```python
from build123d import *

# Parameters (mm, degrees)
SKETCH1_R                   = 6.8
SKETCH1_R_2                 = 4.8
TUBE_SURROUNDING_DEPTH      = 50
FIN_START                   = -100
FIN_HOLDERS_DEPTH           = 100
F_3MM_SUPPORT_FILLETS_R     = 3
F_5MM_FIN_HOLDER_ROUNDING_R = 5


with BuildPart() as part:
    # Sketch1 → Tube surrounding (new, symmetric)
    with BuildSketch(Plane.XY):
        Circle(SKETCH1_R)
        Circle(SKETCH1_R_2, mode=Mode.SUBTRACT)
    extrude(amount=TUBE_SURROUNDING_DEPTH, both=True)

    # Sketch2 → Fin holders (add)
    with BuildSketch(Plane.XY.offset(50).offset(FIN_START)):
        with BuildLine():
            Line((-6.239343856, 2.70380995), (-2.70380995, 6.239343856))
            Line((-2.70380995, 6.239343856), (-8.3606642, 11.896198106))
            Line((-8.3606642, 11.896198106), (-7.300004028, 12.956858277))
            Line((-7.300004028, 12.956858277), (0, 5.656854249))
            Line((0, 5.656854249), (7.300004028, 12.956858277))
            Line((7.300004028, 12.956858277), (8.3606642, 11.896198106))
            Line((8.3606642, 11.896198106), (2.70380995, 6.239343856))
            Line((2.70380995, 6.239343856), (6.239343856, 2.70380995))
            Line((6.239343856, 2.70380995), (11.896198106, 8.3606642))
            Line((11.896198106, 8.3606642), (12.956858277, 7.300004028))
            Line((12.956858277, 7.300004028), (4.704593429, -0.952260821))
            ThreePointArc((4.704593429, -0.952260821), (0, 4.8), (-4.704593429, -0.952260821))
            Line((-4.704593429, -0.952260821), (-12.956858277, 7.300004028))
            Line((-12.956858277, 7.300004028), (-11.896198106, 8.3606642))
            Line((-11.896198106, 8.3606642), (-6.239343856, 2.70380995))
        make_face()
    extrude(amount=FIN_HOLDERS_DEPTH)

    # 3mm support fillets
    # the kernel refuses this fillet: 3 mm, written as the material it adds along each edge
    with BuildSketch(Plane(origin=(1.060017294, 6.716871544, -50), x_dir=(-0.9973250573829818, 0.07309398002593596, 0), z_dir=(0, 0, 1)), Plane(origin=(-6.716871544, 1.060017294, -50), x_dir=(-0.07309398002594036, -0.9973250573829815, 0), z_dir=(0, 0, 1))) as f_3mm_support_fillets_piece_1:
        with BuildLine():
            CenterArc((1.38224034, -2.989581697), F_3MM_SUPPORT_FILLETS_R, 94.776406165, 44.415308597)
            Line((-0.88846134, -1.028991511), (0, 0))
            ThreePointArc((0, 0), (0.566218934, -0.023614819), (1.132437869, 0))
        make_face()
    extrude(amount=100)
    with BuildSketch(Plane(origin=(-1.060017294, 6.716871544, -50), x_dir=(-0.7071067811865461, 0.707106781186549, 0), z_dir=(0, 0, 1)), Plane(origin=(6.716871544, 1.060017294, -50), x_dir=(0.7071067811865486, 0.7071067811865466, 0), z_dir=(0, 0, 1))) as f_3mm_support_fillets_piece_2:
        with BuildLine():
            CenterArc((1.359480446, -3), F_3MM_SUPPORT_FILLETS_R, 90, 44.415308597)
            ThreePointArc((-0.740082191, -0.857142857), (-0.352167026, -0.444004423), (0, 0))
            Line((0, 0), (1.359480446, 0))
        make_face()
    extrude(amount=100)

    # 5mm fin holder rounding
    # the kernel refuses this fillet: 5 mm, written as the material it takes off along each edge
    with BuildSketch(Plane(origin=(12.956858277, 7.300004028, -58.926785536), x_dir=(-0.707106781186548, -0.7071067811865471, 0), z_dir=(0, 0, 1)), Plane(origin=(-7.300004028, 12.956858277, -58.926785536), x_dir=(0.7071067811865471, -0.707106781186548, 0), z_dir=(0, 0, 1))) as f_5mm_fin_holder_rounding_piece_1:
        with BuildLine():
            CenterArc((3.570714214, -5), F_5MM_FIN_HOLDER_ROUNDING_R, 90, 45.572995999)
            Line((0, -1.5), (-0.071414284, -1.43))
            ThreePointArc((-0.071414284, -1.43), (-0.1, -0.75), (-0.1, 0))
            Line((-0.1, 0), (0, 0.1))
            Line((0, 0.1), (3.570714214, 0.1))
            Line((3.570714214, 0.1), (3.570714214, 0))
        make_face()
    extrude(amount=117.853571071, mode=Mode.SUBTRACT)
    with BuildSketch(Plane(origin=(-12.956858277, 7.300004028, -58.926785536), x_dir=(0.7071067811865476, 0.7071067811865476, 0), z_dir=(0, 0, 1))) as f_5mm_fin_holder_rounding_piece_2:
        with BuildLine():
            CenterArc((5, -3.570714214), F_5MM_FIN_HOLDER_ROUNDING_R, 134.427004001, 45.572995999)
            Line((0, -3.570714214), (-0.1, -3.570714214))
            Line((-0.1, -3.570714214), (-0.1, 0))
            Line((-0.1, 0), (0, 0.1))
            ThreePointArc((0, 0.1), (0.75, 0.1), (1.43, 0.071414284))
            Line((1.43, 0.071414284), (1.5, 0))
        make_face()
    extrude(amount=117.853571071, mode=Mode.SUBTRACT)
    with BuildSketch(Plane(origin=(7.300004028, 12.956858277, -58.926785536), x_dir=(-0.707106781186548, -0.707106781186547, 0), z_dir=(0, 0, 1))) as f_5mm_fin_holder_rounding_piece_3:
        with BuildLine():
            CenterArc((3.570714214, 5), F_5MM_FIN_HOLDER_ROUNDING_R, 224.427004001, 45.572995999)
            Line((0, 1.5), (-0.071414284, 1.43))
            ThreePointArc((-0.071414284, 1.43), (-0.1, 0.75), (-0.1, 0))
            Line((-0.1, 0), (0, -0.1))
            Line((0, -0.1), (3.570714214, -0.1))
            Line((3.570714214, -0.1), (3.570714214, 0))
        make_face()
    extrude(amount=117.853571071, mode=Mode.SUBTRACT)


solid = part.part
```
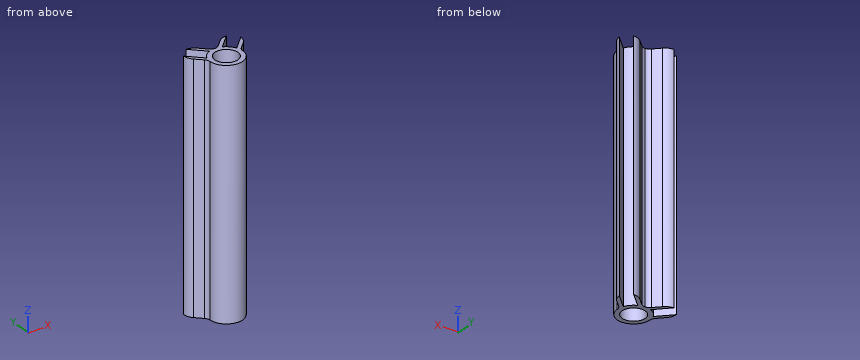
Source: CAD feature listing. Evaluate the final solid. Frame: model axes, mm. Give positions to 0.01 mm unless a question says otherwise; leave off trailing zeros. Loops run counter-clockwise (first coordinate to the right, second up) from the corner with the lowest first, then second, coordinate; pieces in that order, holes last. Notation, with made-up numbers: (21, 14.5) -> (76, 14.5) arc R23 ccw to (76, 39.5) -> close; hole circle Ø1 at (-26, -1). An arc over 180 degrees is marked (long way). Use a Markdown table: item, result. Add a question column.
(1) First-contact query: pin 1 Ø10 at (x, z) = (-9.5, 24.5) entering from -Y; pin 2 Ø3 at (x, z) = (3.5, 24) entering from -Y; pin 3 Ø10 at (y, z) = (-2, 33.5) entering from +X; pin 4 Ø1 at (x, y) = (5, 6.5) entering from +Z. Flat tips, straight axial feed; report the tip coordinate or a pass-through.
(2) Section query B-B (y = -1.75). Output: boundary loops of the cut face in (x, z).
(3) Ray query, line 1 (Y direction, x = 3.5, z = -13); line 2 (X direction, y = 7.75, z = 7); line 3 (X direction, y = 7.5, z = -21.5). Return the intervals inside material, ascending.
(4) Section query A-A (z = 41). Output: boundary loops of the cut face in (x, y).
(5) Section query C-C (x = -9.25). Output: boundary loops of the cut face in (y, z), then the cut area to 3 significant figures.
Checked values:
| question | item | result |
|---|---|---|
| 1 | pin 1 | y = -5.1 |
| 1 | pin 2 | y = -6.5 |
| 1 | pin 3 | x = 8.66 |
| 1 | pin 4 | through |
| 2 | outline | (-6.57, -50) -> (-4.47, -50) -> (-4.47, 50) -> (-6.57, 50) -> close; (4.47, -50) -> (6.57, -50) -> (6.57, 50) -> (4.47, 50) -> close |
| 3 | line 1 | -5.83 to -3.28, 3.28 to 5.83, 7.04 to 9.16 |
| 3 | line 2 | -11.86 to -11.29, -4.21 to -2.09, 2.09 to 4.21, 11.29 to 11.86 |
| 3 | line 3 | -11.83 to -11.04, -3.96 to -1.83, 1.83 to 3.96, 11.04 to 11.83 |
| 4 | outline | (-11.9, 8.36) arc R5 ccw to (-10.43, 4.78) -> (-7.68, 2.02) arc R3 cw to (-6.8, -0.07) arc R6.8 ccw to (6.8, -0.07) arc R3 cw to (7.68, 2.02) -> (10.43, 4.78) arc R5 ccw to (11.9, 8.36) -> (6.24, 2.7) arc R6.8 ccw to (2.7, 6.24) -> (8.36, 11.9) arc R5 ccw to (4.78, 10.43) -> (2.02, 7.68) arc R3 cw to (0, 6.8) arc R3 cw to (-2.02, 7.68) -> (-4.78, 10.43) arc R5 ccw to (-8.36, 11.9) -> (-2.7, 6.24) arc R6.8 ccw to (-6.24, 2.7) -> close; hole circle Ø9.6 at (0, 0) |
| 5 | outline | (3.59, -50) -> (5.71, -50) -> (5.71, 50) -> (3.59, 50) -> close |
| 5 | area | 212 mm^2 |
